The drawing under review shows one solid part. Ordinate dimensions are in mm from its lowest x, y, z. A direction names the side the tool comes from. Coordinates: 2 decimals unless noted, no trailing zeros. Order: outer loops, then holes, each group sorted by start corner. A loop starts at its lowest first (then second) coordinate and runs counter-clockwise, first axis right, second up. Notation, with made-up numbers: (35, -34) - (52, -34) arc R16 ccw to (52, -28) - close; hole circle Ø5 at (-11, 73.25). An arc over 180 degrees is marked (long way). Answer in a Markdown table with one row per item.
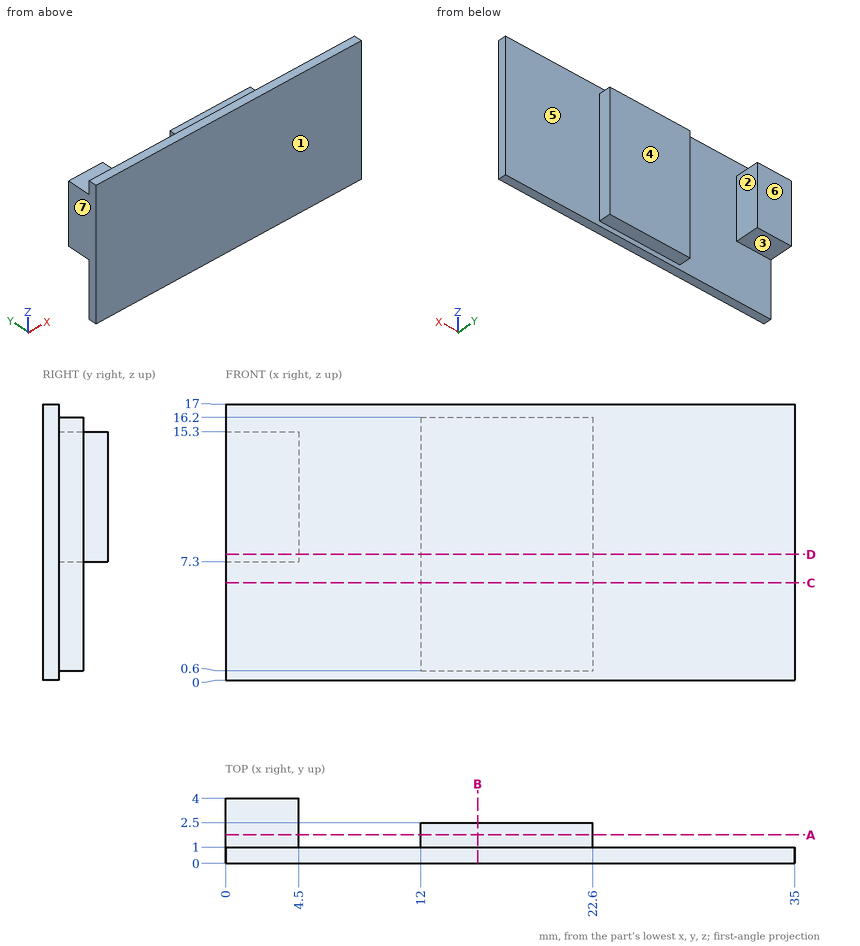
Item 1: We need section C-C, the plane z = 6. Write out the cut boundary in (x, y), then the cut area to 3 significant figures.
Check values:
| item | result |
|---|---|
| outline | (0, 0) - (35, 0) - (35, 1) - (22.6, 1) - (22.6, 2.5) - (12, 2.5) - (12, 1) - (0, 1) - close |
| area | 50.9 mm^2 |
Item 2: To check wall thickness, follow line 1 (X direction, y = 2.2, z = 14.5); line 2 (Y direction, x = 31, z = 10.25); line 3 (Y direction, x = 18, z = 8.75). State the ranges of each line that lie inside material, in increasing order. Write a range as from..to.
Check values:
| item | result |
|---|---|
| line 1 | 0..4.5, 12..22.6 |
| line 2 | 0..1 |
| line 3 | 0..2.5 |
Item 3: Clearance check with flat-ended pins moving along their axes: pin 1 Ø1.2 at (x, y) = (18.5, 2) entering from -Z; pin 2 Ø3 at (x, z) = (19.5, 9.5) entering from +Y; pin 3 Ø1.2 at (y, z) = (2, 11.5) entering from +X. State where each tip first meets the part, or that it passes through.
Check values:
| item | result |
|---|---|
| pin 1 | z = 0.6 |
| pin 2 | y = 2.5 |
| pin 3 | x = 22.6 |
Item 4: We need section A-A, the plane y = 1.75. Write out the cut boundary in (x, z), then the cut area to 3 significant figures.
Check values:
| item | result |
|---|---|
| outline | (0, 7.3) - (4.5, 7.3) - (4.5, 15.3) - (0, 15.3) - close; (12, 0.6) - (22.6, 0.6) - (22.6, 16.2) - (12, 16.2) - close |
| area | 201 mm^2 |
Item 5: Tool access review of the marked faces 1, 2, 3 and 4: name each direction out of +Z, -Z, +X, -X, +Y, -Y from which nothing blocks a thin tool from reaching the whole face with its end or side.
Check values:
| item | result |
|---|---|
| face 1 | +Z, -Z, +X, -X, -Y |
| face 2 | +Z, -Z, +Y |
| face 3 | -Z, -X, +Y |
| face 4 | +Z, -Z, +X, +Y |
Item 6: We need section B-B, the plane x = 15.5. Write out the cut boundary in (y, z).
Check values:
| item | result |
|---|---|
| outline | (0, 0) - (1, 0) - (1, 0.6) - (2.5, 0.6) - (2.5, 16.2) - (1, 16.2) - (1, 17) - (0, 17) - close |
Item 7: We need section D-D, the plane z = 7.75. Write out the cut boundary in (x, y).
Check values:
| item | result |
|---|---|
| outline | (0, 0) - (35, 0) - (35, 1) - (22.6, 1) - (22.6, 2.5) - (12, 2.5) - (12, 1) - (4.5, 1) - (4.5, 4) - (0, 4) - close |
Item 8: Mouldability with a two-part tool opening along X and no side actions: class the marked faces 5, 6 and 7 as +X half, -X half, draft (parallel to the pull), parting line (faces both ways), or undercut.
Check values:
| item | result |
|---|---|
| face 5 | undercut |
| face 6 | draft |
| face 7 | -X half |
